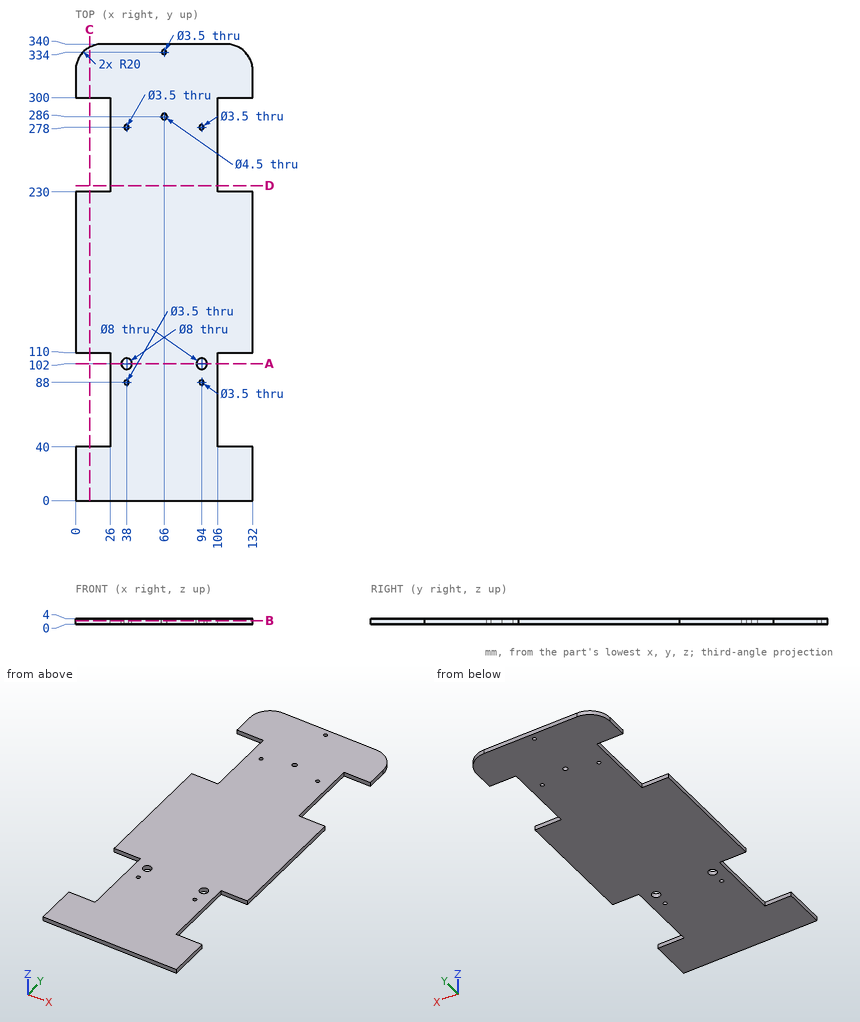
Geometry: see drawing. Coordinates: mm, zero at the bounding-box minimum. Give positions to 0.01 mm unless a question says otherwise; leave off trailing zeros. Loops run counter-clockwise (first coordinate to the right, second up) from the corner with the lowest first, then second, coordinate; pieces in that order, holes last. Notation, with made-up numbers: (71, 2) - (115, 2) arc R12 cw to (115, 6) - close; hole circle Ø9 at (-25.5, 29). An arc over 180 degrees is marked (long way). Use CSV: the item, a comma, the result in double quotes. Start each with the question number.
Item 1: Contact query for a flat-ended pin moving along its axis: P1, Ø5.5, axis at x = 38, y = 88, coming from the +Z side. Output: stop coordinate, or through.
Item 2: Section A-A on y = 102. Return loops of the section in (x, z), then the cut area to 3 significant figures.
Item 3: Line query: line 1 (Y direction, x = 38, z = 1.05); line 2 (Y direction, x = 66, z = 2.2); line 3 (X direction, y = 278, z = 2.65). Output: solid intervals per line, ascending.
Item 4: Section B-B on z = 2.5. State how many separate pieces and enclosed holes the cut face has, then the cut area to 3 significant figures.
Item 5: Section C-C on x = 10.5. Return loops of the section in (y, z).
Item 6: Section D-D on y = 234.5. Return loops of the section in (x, z), then the cut area to 3 significant figures.
Ans:
1,P1,"stops at z = 4"
2,outline,"(26, 0) - (34, 0) - (34, 4) - (26, 4) - close; (42, 0) - (90, 0) - (90, 4) - (42, 4) - close; (98, 0) - (106, 0) - (106, 4) - (98, 4) - close"
2,area,"256 mm2"
3,line 1,"y = 0 to 86.25, 89.75 to 98, 106 to 276.25, 279.75 to 340"
3,line 2,"y = 0 to 283.75, 288.25 to 332.25, 335.75 to 340"
3,line 3,"x = 26 to 36.25, 39.75 to 92.25, 95.75 to 106"
4,separate pieces,"1"
4,enclosed holes,"8"
4,area,"37,300 mm2"
5,outline,"(0, 0) - (40, 0) - (40, 4) - (0, 4) - close; (110, 0) - (230, 0) - (230, 4) - (110, 4) - close; (300, 0) - (337.6, 0) - (337.6, 4) - (300, 4) - close"
6,outline,"(26, 0) - (106, 0) - (106, 4) - (26, 4) - close"
6,area,"320 mm2"
